The model under review builds one solid part; all positions refer to its coordinate system, in mm. A direction names the side the tool comes from. Round coordinates to 2 decimals unless told otherwise and drop trailing zeros. Write each loop counter-clockwise with the first axis right and the second up, starting at its lowest first coordinate (ties: lowest second). Pieces come first, ordered by that corner, then holes. Notation, with made-up numbers: M 33,2.25 L 76,2.25 A26 cw 76,39.25 Z; hole C -3.5,-38.5 d7. An arc over 180 degrees is marked long. Write item = value, one per line. Start each with the question number.
Item 1: Tool access review of faces 4 (the flat face through (103, 17, 0)), 5 (the flat face through (53, 14, 20.5)), 6 (the flat face through (19, 41, 0)): name each direction out of +Z, -Z, +X, -X, +Y, -Y from which nothing blocks a thin tool from reaching the whole face with its end or side.
Item 2: To check wall thickness, follow line 1 along X through (y, z) = (3, -3); line 2 along Y through (x, z) = (17, 9); line 3 along Y through (x, z) = (30, 20). State the ranges of each line that lie inside material, in increasing order.
Item 3: Take a section at A-A, the plane z = -1. Give the boundary of the cut face in (x, y), plus the area to 3 significant figures.
Item 4: For pin 1 Ø8.5 at (x, y) = (50, 21.5) entering from +Z; pin 2 Ø6 at (y, z) = (17.5, -9.5) entering from +X; pin 3 Ø6.5 at (x, z) = (106.5, 1.5) entering from +Y; pin 4 Ø12 at (x, y) = (46.5, 39.5) entering from +Z, all flat-tipped, find the tip position at first contact; note any pin that passes through.
Item 5: The part is to be moulded in two halves that separate along Z. For faces 1 (the flat face through (5, 26, -19)), 2 (the flat face through (53, 14, -20.5)), 3 (the flat face through (28, 31, 0)), say which applies: +Z half, -Z half, draft (parallel to the pull), parting line (faces both ways), or undercut.
Item 6: Take a section at D-D, the plane x = 59. Give the boundary of the cut face in (y, z).
Item 7: Take a section at B-B, the plane y = 31. Give the boundary of the cut face in (x, z), plus the area to 3 significant figures.
Item 8: Take a section at C-C, the plane y = 19.5. Give the boundary of the cut face in (x, z), plus the area to 3 significant figures.
from build123d import *

# Parameters (mm, degrees)
BOSS_EXTRUDE1_DEPTH   = 52
BOSS_EXTRUDE1_2_DEPTH = 52
SKETCH1_3_W           = 18
SKETCH1_3_H           = 23
BOSS_EXTRUDE2_DEPTH   = 41
BOSS_EXTRUDE3_DEPTH   = 29
BOSS_EXTRUDE4_DEPTH   = 17
SKETCH2_R             = 5.5
CUT_EXTRUDE1_DEPTH    = 30.5


with BuildPart() as part:
    # Sketch1 → Boss-Extrude1 (new body)
    with BuildSketch(Plane(origin=(0, 0, 0), x_dir=(1, 0, 0), z_dir=(0, 1, 0))):
        Polygon((28, -11.5), (10, -11.5), (10, -19), (0, -19), (0, -30.5), (28, -30.5), (28, -20.5), align=None)
    extrude(amount=BOSS_EXTRUDE1_DEPTH)



with BuildPart() as body_2:
    # Sketch1 → Boss-Extrude1 2 (new body)
    with BuildSketch(Plane(origin=(0, 0, 0), x_dir=(1, 0, 0), z_dir=(0, 1, 0))):
        Polygon((0, 19), (10, 19), (10, 11.5), (28, 11.5), (28, 20.5), (28, 30.5), (0, 30.5), align=None)
    extrude(amount=BOSS_EXTRUDE1_2_DEPTH)


with BuildPart() as part_1:
    add(part.part)

    add(body_2.part)  # Boss-Extrude2 merges body 2
    # Sketch1_3 → Boss-Extrude2 (add)
    with BuildSketch(Plane(origin=(0, 0, 0), x_dir=(1, 0, 0), z_dir=(0, 1, 0))):
        with Locations((19, 0)):
            Rectangle(SKETCH1_3_W, SKETCH1_3_H)
    extrude(amount=BOSS_EXTRUDE2_DEPTH)

    # Sketch1_4 → Boss-Extrude3 (add)
    with BuildSketch(Plane(origin=(0, 0, 0), x_dir=(1, 0, 0), z_dir=(0, 1, 0))):
        Polygon((28, 20.5), (28, 11.5), (28, -11.5), (28, -20.5), (77.968771248, -20.5), (98, -10.730116948), (98, 10.730116948), (77.968771248, 20.5), align=None)
    extrude(amount=BOSS_EXTRUDE3_DEPTH)

    # Sketch1_5 → Boss-Extrude4 (add)
    with BuildSketch(Plane(origin=(0, 0, 0), x_dir=(1, 0, 0), z_dir=(0, 1, 0))):
        Polygon((110.968771248, 4.404824577), (98, 10.730116948), (98, -10.730116948), (110.968771248, -4.404824577), align=None)
    extrude(amount=BOSS_EXTRUDE4_DEPTH)

    # Sketch2 → Cut-Extrude1 (cut, symmetric)
    with BuildSketch(Plane.XY):
        with Locations(Location((77.968771248, 17, 0), (0, 0, 270))):
            Circle(SKETCH2_R)
    extrude(amount=CUT_EXTRUDE1_DEPTH, both=True, mode=Mode.SUBTRACT)


solid = part_1.part
Response values:
q1.face_4 = +Z, -Z, +X, +Y
q1.face_5 = +Z, +X, +Y, -Y
q1.face_6 = +X, -X, +Y
q2.line_1 = 10 to 110.97
q2.line_2 = 0 to 41
q2.line_3 = 0 to 29
q3.outline = M 10,0 L 110.97,0 L 110.97,17 L 98,17 L 98,29 L 28,29 L 28,41 L 10,41 Z; hole C 77.97,17 d11
q3.area = 2,890 mm2
q4.pin_1 = 20.5
q4.pin_2 = 106.59
q4.pin_3 = 17
q4.pin_4 = through
q5.face_1 = undercut
q5.face_2 = -Z half
q5.face_3 = draft
q6.outline = M 0,-20.5 L 29,-20.5 L 29,20.5 L 0,20.5 Z
q7.outline = M 0,-30.5 L 28,-30.5 L 28,30.5 L 0,30.5 L 0,19 L 10,19 L 10,-19 L 0,-19 Z
q7.area = 1,330 mm2
q8.outline = M 0,-30.5 L 28,-30.5 L 28,-20.5 L 73.07,-20.5 L 73.07,20.5 L 28,20.5 L 28,30.5 L 0,30.5 L 0,19 L 10,19 L 10,-19 L 0,-19 Z; M 82.87,-18.11 L 98,-10.73 L 98,10.73 L 82.87,18.11 Z
q8.area = 3,610 mm2
